Check sheet for the drawn part. Datum: minimum x, y, z corner. Units: mm. A direction names the side the tool comes from. Round coordinates to 2 decimals unless told otherwise and drop trailing zeros. Order: outer loops, then holes, each group sorted by start corner. A loop starts at its lowest first (then second) coordinate and runs counter-clockwise, first axis right, second up. Notation, with made-up numbers: M 67.25,-40 L 118.25,-40 A20 cw 118.25,-26 Z; hole C 11.25,10.25 d2. An arc over 180 degrees is marked long. Write item = value, one per line. Start each with the question number.
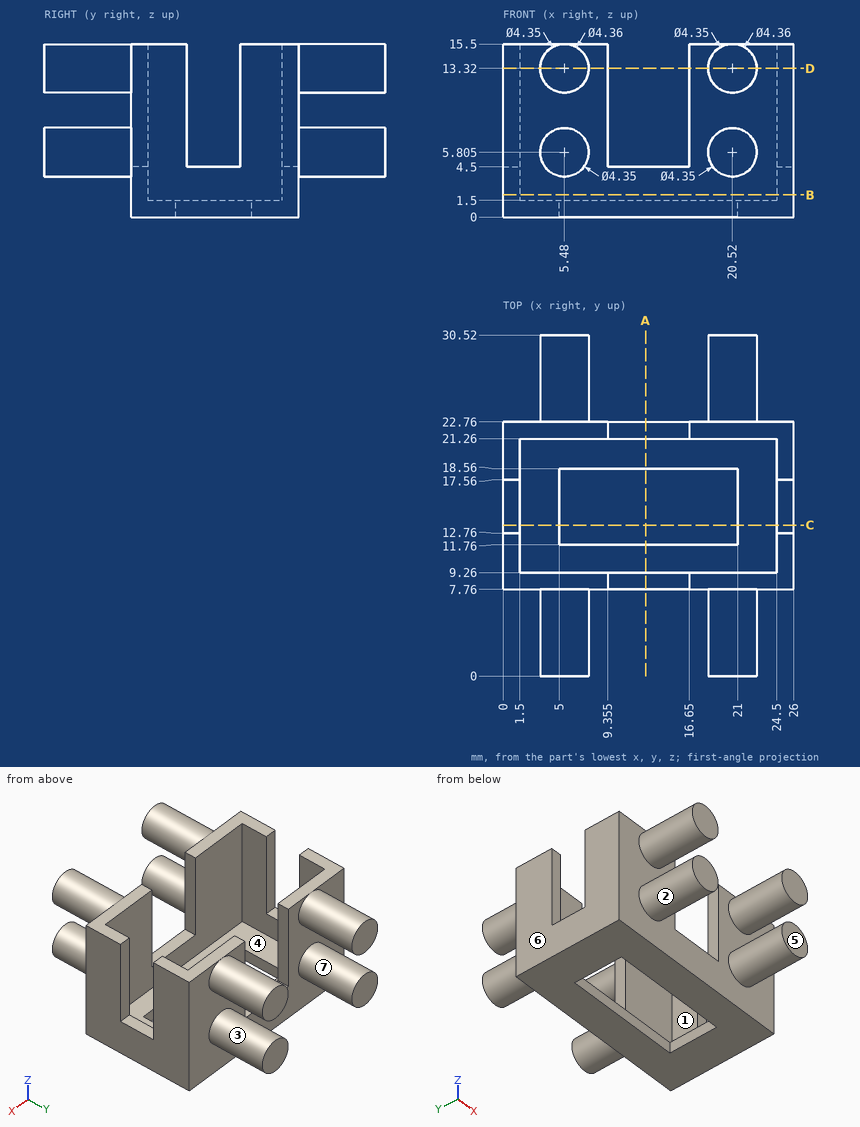
1) Cross-section at A-A, the plane x = 12.75. Enter the section's corners in (y, z).
2) Cross-section at D-D, the plane z = 13.32. Give the number of separate pieces and of enclosed holes in the cut face, then the cut area to 3 significant figures.
3) Cross-section at B-B, the plane z = 2. Enter the section's corners in (x, y).
4) Cross-section at C-C, the plane y = 13.5. Enter the section's corners in (x, z).
5) Gauge pin test, flat ends, axial feed: P1, Ø1.2, axis at x = 15, z = 0.5, coming from the -Y side; P2, Ø1.6, axis at x = 25.5, y = 15.5, coming from the +Z side. Record the tip position at first contact, or that the pin passes through.
6) Access from +Z, -Z, +X, -X, +Y, -Y to the whole of each face (thin tool, end or side, straight path). Record for the marked faces 1, 2 and 3.
7) Release check for a two-part mould opening along X. For the marked faces 4, 5, 6 and 7 record: pulls with the +X half, pulls with the -X half, needs draft (parallel to the pull), parting line crosses it, or undercut.
8) Scan lines: probe 1 along Y at (x, z) = (9.5, 1.25); probe 2 along Y at (x, z) = (13.5, 3); probe 3 along X at (y, z) = (22.5, 9.25) (3 decimals). Record each from-to range of solid material in increasing order.
Geometry results:
q1.outline = M 7.76,0 L 11.76,0 L 11.76,1.5 L 9.26,1.5 L 9.26,4.5 L 7.76,4.5 Z; M 18.56,0 L 22.76,0 L 22.76,4.5 L 21.26,4.5 L 21.26,1.5 L 18.56,1.5 Z
q2.separate_pieces = 4
q2.enclosed_holes = 0
q2.area = 213 mm^2
q3.outline = M 0,7.76 L 26,7.76 L 26,22.76 L 0,22.76 Z; hole M 1.5,9.26 L 24.5,9.26 L 24.5,21.26 L 1.5,21.26 Z
q4.outline = M 0,0 L 5,0 L 5,1.5 L 1.5,1.5 L 1.5,4.5 L 0,4.5 Z; M 21,0 L 26,0 L 26,4.5 L 24.5,4.5 L 24.5,1.5 L 21,1.5 Z
q5.P1 = 7.76
q5.P2 = 4.5
q6.face_1 = +Z
q6.face_2 = -Y
q6.face_3 = +Y
q7.face_4 = undercut
q7.face_5 = needs draft
q7.face_6 = pulls with the -X half
q7.face_7 = undercut
q8.probe_1 = 7.76 to 11.76, 18.56 to 22.76
q8.probe_2 = 7.76 to 9.26, 21.26 to 22.76
q8.probe_3 = 0 to 9.355, 16.65 to 26
